Geometry check sheet. Reference: the model listing, model coordinates, mm. A direction names the side the tool comes from. Give positions to 0.01 mm unless a question says otherwise; leave off trailing zeros. Write each loop counter-clockwise with the first axis right and the second up, starting at its lowest first coordinate (ties: lowest second). Pieces come first, ordered by that corner, then holes.
(1) Thickness scan on line 1 along Y through (x, z) = (14.4, 7.75); line 2 along Z through (x, y) = (18, -9.25); line 3 along Y through (x, z) = (27, 3.75). Record the ranges inside material, lowest first.
(2) Cross-section at C-C (z = 7.25). Record the boundary of the cut face in (x, y).
(3) Mould release check, pull along X, two halves, no side actions. Record for faces 1 (the cylindrical face through (28.61, 4.48, 5.28)), 2 (the cylindrical face through (-0.6, 0, -0.5)), 3 (the flat face through (11, 0, 10.6)): +X half, -X half, draft (parallel to the pull), parting line (faces both ways), or undercut.
(4) Depth check by flat-ended pin: P1, Ø1.5, axis at y = -5.5, z = 0.5, coming from the -X side; P2, Ø3, axis at x = 5.5, z = 6, coming from the +Y side. Enter the tip coordinate at first touch or a pass-through.
(5) Cross-section at A-A (x = 14.4). Record the boundary of the cut face in (y, z), and give its area (3 significant figures).
(6) Tool access check on faces 4 (the cylindrical face through (29.354, -0.23, -0.508)), 5 (the cylindrical face through (16.83, 0.77, 5.03)). Record the directions out of +Z, -Z, +X, -X, +Y, -Y that give a thin tool (end or side, any length) a straight path to the whole face; none if there is none.
```python
from build123d import *

# Parameters (mm, degrees)
SKETCH_R          = 14.9
SKETCH_R_2        = 2.55
PAD_DEPTH         = 10.5
FILLET_R          = 0.5
SKETCH001_R       = 0.6
PAD001_DEPTH      = 5.25
PAD001_DEPTH_BACK = 3.5


with BuildPart() as fillet_body:
    # Sketch → Pad (new body)
    with BuildSketch(Plane.XY.offset(0.1)):
        with Locations((14.4, 0)):
            Circle(SKETCH_R)
        with Locations((14.4, 0)):
            Circle(SKETCH_R_2, mode=Mode.SUBTRACT)
    extrude(amount=PAD_DEPTH)

    # Fillet
    fillet_edges = [fillet_body.edges().sort_by_distance(p)[0] for p in [
        (11.85, 0, 10.6),
        (-0.5, 0, 10.6),
        (-0.5, 0, 0.1),
    ]]
    fillet(fillet_edges, radius=FILLET_R)


with BuildPart() as obj1:
    # Sketch001 → Pad001 (new body, two sides)
    with BuildSketch(Plane.XY.offset(0.5)) as pad001_sk:
        Circle(SKETCH001_R)
        with Locations((28.8, 0)):
            Circle(SKETCH001_R)
    extrude(amount=PAD001_DEPTH)
    extrude(pad001_sk.sketch, amount=-PAD001_DEPTH_BACK)

    # obj1: union Fillet body
    add(fillet_body.part)


solid = obj1.part
```
Reply:
1. line 1: y = -14.9 to -2.55, 2.55 to 14.9
1. line 2: z = 0.1 to 10.6
1. line 3: y = -7.95 to 7.95
2. outline: circle Ø29.8 at (14.4, 0); hole circle Ø5.1 at (14.4, 0)
3. face 1: parting line
3. face 2: undercut
3. face 3: draft
4. P1: stops at x = 0.28
4. P2: stops at y = 12.93
5. outline: (-14.9, 0.6) arc R0.5 ccw to (-14.4, 0.1) - (-2.55, 0.1) - (-2.55, 10.1) arc R0.5 ccw to (-3.05, 10.6) - (-14.4, 10.6) arc R0.5 ccw to (-14.9, 10.1) - close; (2.55, 0.1) - (14.4, 0.1) arc R0.5 ccw to (14.9, 0.6) - (14.9, 10.1) arc R0.5 ccw to (14.4, 10.6) - (3.05, 10.6) arc R0.5 ccw to (2.55, 10.1) - close
5. area: 259 mm2
6. face 4: -Z
6. face 5: +Z, -Z
